Here's the drawing with two shaded views (mm, measured from the low corner). I have some questions. A direction names the side the tool comes from. Give positions to 0.01 mm unless a question says otherwise; leave off trailing zeros. Write each loop counter-clockwise with the first axis right and the second up, starting at its lowest first coordinate (ties: lowest second). Pieces come first, ordered by that corner, then holes. Notation, with made-up numbers: (23, 19.5) -> (66, 19.5) arc R14 ccw to (66, 42.5) -> close; hole circle Ø1 at (22, 52). An arc over 180 degrees is marked (long way). One line per item, written item: value.
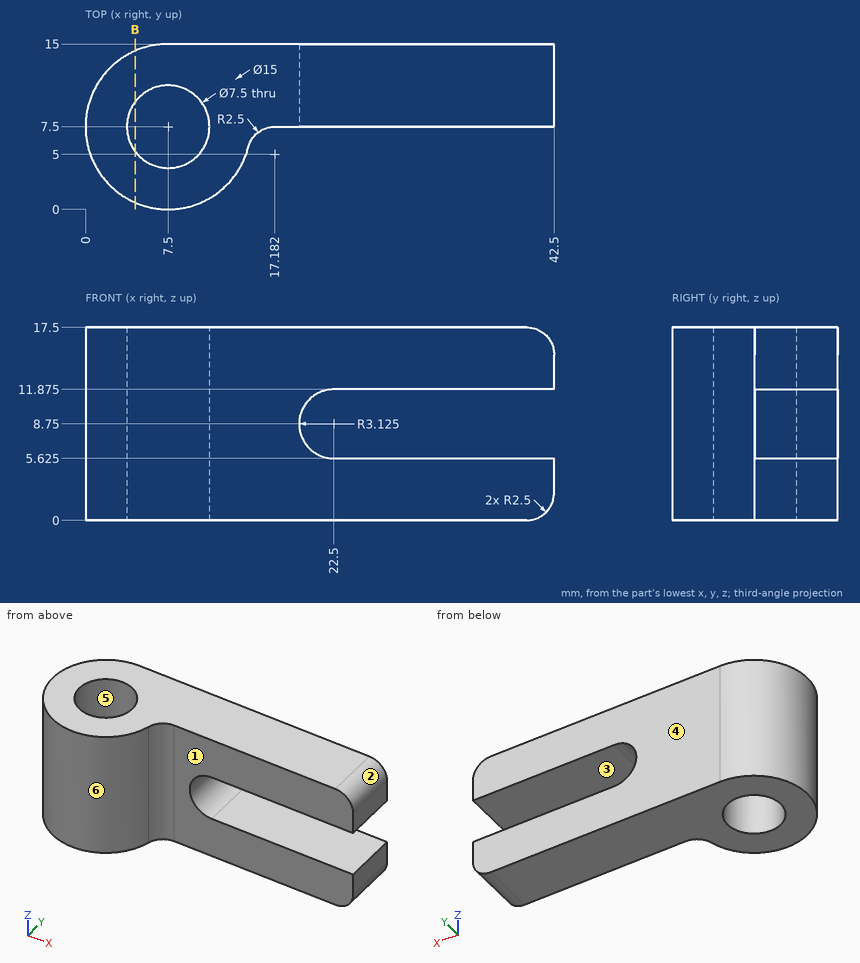
1) For the marked faces 1, 2 and 3, which set-ups out of +Z, -Z, +X, -X, +Y, -Y let a thin tool reach every point of the face, with its end or its side?
Answer list:
face 1: +Z, -Z, +X, -Y
face 2: +Z, +X, +Y, -Y
face 3: +X, +Y, -Y
2) Will these pins go through, and if not, where does the flat tip stop? pin 1 (5 mm diameter, centred on y = 3, z = 3, fed in from -X); pin 2 (5 mm diameter, centred on x = 34, z = 9.5, fed in from -Y); pin 3 (5 mm diameter, centred on y = 12.5, z = 12.5, fed in from -X).
Answer list:
pin 1: stops at x = 0.27
pin 2: stops at y = 7.5
pin 3: stops at x = 0.43
3) I need wall thicknesses on L1, parallel to X at y = 7.75, z = 3 (1 decimal); L2, parallel to X at y = 5.5, z = 11.25; L3, parallel to Z at x = 41, y = 14.25 (1 decimal). Which ranges of each line are inside material? Lowest first, please.
Answer list:
L1: x = 0 to 3.8, 11.2 to 42.5
L2: x = 0.27 to 4.33, 10.67 to 14.73
L3: z = 0.2 to 5.6, 11.9 to 17.3
4) If we section it at B-B (x = 4.5): Write out the boundary of the cut face in (y, z), and give its area (3 significant figures).
Answer list:
outline: (0.63, 0) -> (5.25, 0) -> (5.25, 17.5) -> (0.63, 17.5) -> close; (9.75, 0) -> (14.37, 0) -> (14.37, 17.5) -> (9.75, 17.5) -> close
area: 162 mm^2
5) We'd pull the mould along Y, two halves only. Please class the marked faces 4, 5 and 6: released by +Y, released by -Y, zero draft, split by the parting line, or undercut.
Answer list:
face 4: released by +Y
face 5: undercut
face 6: split by the parting line
